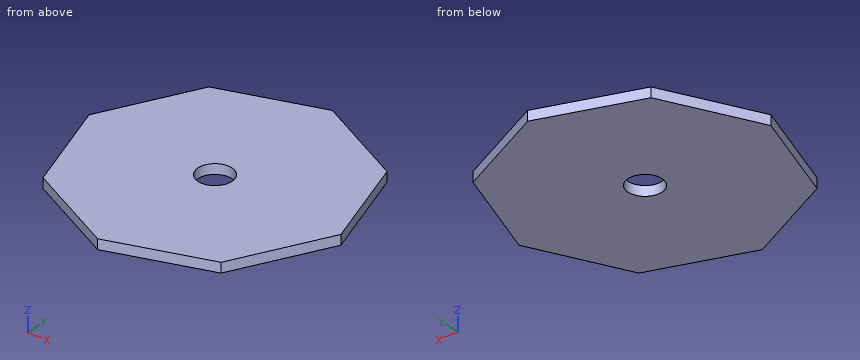
```python
from build123d import *

# Parameters (mm, degrees)
F1_DEPTH = 6.35
F2_R     = 10.922
F3_DEPTH = 25.4


with BuildPart() as f1:
    # F0 (on Top) → F1 (new body)
    with BuildSketch(Plane.XY):
        Polygon((-58.525931, 64.586785), (-87.053837, 4.285671), (-64.586785, -58.525931), (-4.285671, -87.053837), (58.525931, -64.586785), (87.053837, -4.285671), (64.586785, 58.525931), (4.285671, 87.053837), align=None)
    extrude(amount=F1_DEPTH)

    # F2 (on face) → F3 (cut)
    with BuildSketch(Plane.XY.offset(6.35)):
        Circle(F2_R)
    extrude(amount=-F3_DEPTH, mode=Mode.SUBTRACT)


solid = f1.part
```
Geometry check sheet. Reference: the model listing, model coordinates, mm. Coordinates: 2 decimals unless noted, no trailing zeros. Write each loop counter-clockwise with the first axis right and the second up, starting at its lowest first coordinate (ties: lowest second). Pieces come first, ordered by that corner, then holes. Notation, with made-up numbers: M 9.25,-32 L 44.25,-32 A16 cw 44.25,-22 Z; hole C 22,39.5 d1. An arc over 180 degrees is marked long. One line per item, written item: value. Start each with the question number.
(1) Depth check by flat-ended pin: pin 1 (1.5 mm diameter, centred on x = 41, z = 1, fed in from -Y); pin 2 (2 mm diameter, centred on x = 6, z = 1, fed in from -Y); pin 3 (2 mm diameter, centred on y = -58.5, z = 1.5, fed in from -X); pin 4 (25 mm diameter, centred on x = 0, y = 0, fed in from -Z). Enter the tip coordinate at first touch or a pass-through.
(2) Sectioned sample at B-B, the plane y = 0. Enter the section's corners in (x, z), and give its area (3 significant figures).
(3) Scan lines: line 1 along Y through (x, z) = (0, 2); line 2 along Y through (x, z) = (6.5, 5.25); line 3 along Y through (x, z) = (-49, 4.5). Record each from-to range of solid material in increasing order. Write a range as [from, to].
(4) Sectioned sample at A-A, the plane z = 1.5. Enter the section's corners in (x, y).
(5) Sectioned sample at D-D, the plane x = -75. Enter the section's corners in (y, z).
Filled sheet:
1. pin 1: y = -71.12
1. pin 2: y = -83.73
1. pin 3: x = -64.95
1. pin 4: z = 0
2. outline: M -85.52,0 L -10.92,0 L -10.92,6.35 L -85.52,6.35 Z; M 10.92,0 L 85.52,0 L 85.52,6.35 L 10.92,6.35 Z
2. area: 947 mm²
3. line 1: [-85.52, -10.92], [10.92, 85.52]
3. line 2: [-83.2, -8.78], [8.78, 86.01]
3. line 3: [-65.9, 67.99]
4. outline: M -87.05,4.29 L -64.59,-58.53 L -4.29,-87.05 L 58.53,-64.59 L 87.05,-4.29 L 64.59,58.53 L 4.29,87.05 L -58.53,64.59 Z; hole C 0,0 d21.84
5. outline: M -29.41,0 L 29.76,0 L 29.76,6.35 L -29.41,6.35 Z
